Autodesk Fusion 360 part; units mm, degrees
sketch "Sketch1" plane through (0, 0, 0) normal (0, 1, 0) x (1, 0, 0)
  line L0 (0, 0) -> (8.5, 0)
  line L1 (0, 0) -> (0, -70)
  line L2 (8.5, 0) -> (8.5, -7)
  line L3 (8.5, -7) -> (8, -7)
  line L4 (8, -7) -> (8, -8.5)
  line L5 (8.5, -7) -> (0, -7)
  line L6 (8, -8.5) -> (0, -8.5)
  line L7 (0, -8.5) -> (0, -15.5)
  line L8 (0, -15.5) -> (4, -15.5)
  arc A0 (8, -8.5) -> (4, -15.5) centre (8, -13.1429) ccw
  line L9 (4, -15.5) -> (4, -17.5)
  line L10 (4, -17.5) -> (0, -17.5)
  line L11 (0, -17.5) -> (4.5, -17.5)
  line L12 (0, -17.5) -> (0, -27)
  line L13 (0, -27) -> (8.5, -27)
  arc A1 (8.5, -27) -> (4.5, -17.5) centre (0.9117, -24.603) ccw
  line L14 (0, -27) -> (0, -51.5)
  line L15 (0, -51.5) -> (4, -51.5)
  arc A2 (8.5, -27) -> (4, -51.5) centre (33.8925, -44.3272) ccw
  line L16 (0, -51.5) -> (3.5, -51.5)
  line L17 (3.5, -51.5) -> (3.5, -53.5)
  line L18 (3.5, -53.5) -> (0, -53.5)
  line L19 (0, -53.5) -> (4, -53.5)
  line L20 (0, -53.5) -> (0, -59.5)
  line L21 (0, -59.5) -> (8.5, -59.5)
  arc A3 (4, -53.5) -> (8.5, -59.5) centre (10.7181, -53.1489) ccw
  line L22 (0, -59.5) -> (0, -61)
  line L23 (0, -61) -> (8, -61)
  line L24 (0, -61) -> (7, -61)
  line L25 (7, -61) -> (7, -63)
  line L26 (7, -63) -> (0, -63)
  line L27 (0, -63) -> (8.5, -63)
  line L28 (8.5, -63) -> (8.5, -70)
  line L29 (8.5, -70) -> (0, -70)
  arc A4 (8, -61) -> (8.5, -59.5) centre (7.0099, -59.8366) ccw
  dimension "d2" = 70
  dimension "d3" = 7
  dimension "d5" = 1.5
  dimension "d7" = 7
  dimension "d12" = 2
  dimension "d15" = 9.5
  dimension "d17" = 24.5
  dimension "d20" = 2
  dimension "d22" = 6
  dimension "d24" = 1.5
  dimension "d26" = 2
  dimension "d29" = 7
revolve "Revolve1" add sketch "Sketch1" angle 360 about axis through (0, 0, 0) along (0, 0, 1)
Input: part model. Units: mm. Frame: model coordinates. A direction names the side the tool comes from. Coordinates: 2 decimals unless noted, no trailing zeros. Loops run counter-clockwise (first coordinate to the right, second up) from the corner with the lowest first, then second, coordinate; pieces in that order, holes last. Notation, with made-up numbers: M -40,66 L -15,66 A26 cw -15,83 Z; hole C 12.5,-28.5 d8. An arc over 180 degrees is marked long. One line per item, written item: value.
(1) Line query: line 1 along Z through (x, y) = (-3.75, 2.75); line 2 along Z through (x, y) = (-0.5, 5.75); line 3 along Z through (x, y) = (-7, 4.5). Output: solid intervals per line, ascending. Write a range as from..to.
Filled in:
line 1: 0..9.93, 17.58..34.85, 56.05..70
line 2: 0..9.07, 18.3..31.91, 57.71..70
line 3: 0..7, 21.7..27.26, 59.43..60.62, 63..70
(2) Pin query (flat end, axial travel): pin 1 (3 mm diameter, centred on x = 4, y = 4, fed in from -Z); pin 2 (2 mm diameter, centred on x = 7, z = 16.5, fed in from -Y); pin 3 (5 mm diameter, centred on x = -5.5, z = 22, fed in from +Y); pin 4 (6 mm diameter, centred on y = 6.5, z = 52, fed in from -X). Return the tip coordinate at first contact, or that it passes through.
Filled in:
pin 1: z = 0
pin 2: through
pin 3: y = 8.1
pin 4: x = -1.86
(3) Section A-A (y = 6). Give the number of separate pieces and of enclosed holes in the cut face, and give its area (3 significant figures).
Filled in:
separate pieces: 3
enclosed holes: 0
area: 356 mm^2
(4) Section B-B (z = 31.5). Output: boundary loops of the cut face in (x, y).
Filled in:
outline: C 0,0 d11.91
(5) Reachability of faces 4 (the cylindrical face through (4.57, 7.167, 3.549)), 5 (the cylindrical face through (-0.867, -3.905, 16.514)), 6 (the flat face through (0, 0, 0)) from +Z, -Z, +X, -X, +Y, -Y: full face, straight path, thin tool, end or side. Return the list, or none.
Filled in:
face 4: -Z
face 5: none
face 6: -Z, +X, -X, +Y, -Y
(6) Pull-direction query (Z, two-part tool) for faces 1 (the flat face through (-3, -3, 17.5)), 2 (the flat face through (0, 0, 70)), 3 (the cylindrical face through (4.57, 7.167, 66.549)); classes: +Z half, -Z half, draft (parallel to the pull), parting line (faces both ways), or undercut.
Filled in:
face 1: undercut
face 2: +Z half
face 3: draft
(7) Section C-C (z = 57). Output: boundary loops of the cut face in (x, y), and give its area (3 significant figures).
Filled in:
outline: C 0,0 d10.4
area: 85.0 mm^2
